Here's how the part is built. I have some questions about the finished solid (model axes, mm). A direction names the side the tool comes from. Give positions to 0.01 mm unless a question says otherwise; leave off trailing zeros. Loops run counter-clockwise (first coordinate to the right, second up) from the corner with the lowest first, then second, coordinate; pieces in that order, holes last. Notation, with made-up numbers: M 79.5,88.5 L 89.5,88.5 A22 cw 89.5,108.5 Z; hole C -20,-15.75 d1. An arc over 180 degrees is marked long. Answer as CSV lines item,"result". Start each with the question number.
Item 1: For faces 1 (the flat face through (-5.8, 0, 7.7)), 2 (the flat face through (8, -10, 18)), 3 (the cylindrical face through (1.22, -7.66, 6.31)), which set-ups out of +Z, -Z, +X, -X, +Y, -Y let a thin tool reach every point of the face, with its end or its side?
Item 2: Will these pins go through, and if not, where does the flat tip stop? P1, Ø2, axis at y = -6.5, z = 19.5, coming from the +X side; P2, Ø3, axis at x = 0.03, y = -8.03, coming from the -Z side; P3, Ø6, axis at y = -8, z = 15, coming from the -X side; P4, Ø10, axis at x = -4, y = 1.5, coming from the -Z side.
Item 3: I want a section at B-B on y = 4. List the corners of the cut face in (x, z) for me.
Item 4: I want a section at C-C on x = 0. List the corners of the cut face in (y, z) for me.
Item 5: I want a section at A-A on z = 15. List the corners of the cut face in (x, y) for me.
Item 6: If we mould it in two halves opening along Z, with no side actions, what happens to faces 4 (the cylindrical face through (-2.38, 0.51, 4.26)), 5 (the flat face through (3, 9, 7)), 6 (the cylindrical face through (-1.788, -0.367, 6.946))? For each: released by +Z, released by -Z, zero draft, split by the parting line, or undercut.
Item 7: I want a section at D-D on y = -5.75. List the corners of the cut face in (x, z) for me.
Item 8: If I drill on line 1 along Z through (x, y) = (-5.5, -7.5); line 2 along X through (y, z) = (5.25, 8.75); line 3 along Z through (x, y) = (0, 7), over which ranges is the centre line in solid material (lowest first)? Write a range as from..to.
from build123d import *

# Parameters (mm, degrees)
SKETCH010_R      = 11
SKETCH010_R_2    = 8.25
PAD005_DEPTH     = 19
SKETCH011_R      = 11.25
SKETCH011_R_2    = 9.25
POCKET005_DEPTH  = 10
CHAMFER003_SIZE2 = 2
CHAMFER003_SIZE  = 8
SKETCH012_R      = 1.25
HOLE_DEPTH       = 25


with BuildPart() as part:
    # Sketch010 → Pad005 (new body)
    with BuildSketch(Plane.XZ.offset(-10)):
        with Locations((0, 15)):
            Circle(SKETCH010_R)
        with Locations((0, 15)):
            Circle(SKETCH010_R_2, mode=Mode.SUBTRACT)
    extrude(amount=PAD005_DEPTH)

    # Sketch011 → Pocket005 (cut)
    with BuildSketch(Plane.XZ.offset(9)):
        with Locations((0.134772, 15)):
            Circle(SKETCH011_R)
        with Locations((0.134772, 15)):
            Circle(SKETCH011_R_2, mode=Mode.SUBTRACT)
    extrude(amount=-POCKET005_DEPTH, mode=Mode.SUBTRACT)

    # Chamfer003
    chamfer003_edges = [part.edges().sort_by_distance(p)[0] for p in [
        (-11, 10, 15),
    ]]
    chamfer003_side = part.faces().sort_by_distance((-11, 5.5, 15))[0]
    chamfer(chamfer003_edges, length=CHAMFER003_SIZE, length2=CHAMFER003_SIZE2, reference=chamfer003_side)

    # Sketch012 → Hole (cut)
    with BuildSketch(Plane.XY.offset(7)):
        with Locations((0.028156, -7.033275)):
            Circle(SKETCH012_R)
    extrude(amount=-HOLE_DEPTH, mode=Mode.SUBTRACT)


with BuildPart() as part_1:
    # Body006 placement: moved
    add(part.part.moved(Location((0, -1, 0))))


solid = part_1.part
Result:
1,face 1,"-Y"
1,face 2,"+Z, -Z, +X, -X, -Y"
1,face 3,"-Z"
2,P1,"x = 8.7"
2,P2,"z = 5.75"
2,P3,"x = -9.12"
2,P4,"z = 4"
3,outline,"C 0,15 d20.5; hole C 0,15 d16.5"
4,outline,"M -10,5.75 L -9.28,5.75 L -9.28,6.75 L -10,6.75 Z; M -10,23.25 L 9,23.25 L 9,24 L 1,26 L 0,26 L 0,24.25 L -10,24.25 Z; M -6.78,5.75 L 0,5.75 L 0,4 L 1,4 L 9,6 L 9,6.75 L -6.78,6.75 Z"
5,outline,"M -11,0 L -9.12,0 L -9.12,-10 L -8.25,-10 L -8.25,9 L -9,9 L -11,1 Z; M 8.25,-10 L 9.38,-10 L 9.38,0 L 11,0 L 11,1 L 9,9 L 8.25,9 Z"
6,face 4,"split by the parting line"
6,face 5,"zero draft"
6,face 6,"undercut"
7,outline,"C 0.13,15 d18.5; hole C 0,15 d16.5"
8,line 1,"7.66..8.85, 21.15..22.34"
8,line 2,"-7.73..-5.39, 5.39..7.73"
8,line 3,"5.5..6.75, 23.25..24.5"
